Can you work these out from the model? Positions are in its coordinate system, mm. Coordinates: 2 decimals unless noted, no trailing zeros. Loops run counter-clockwise (first coordinate to the right, second up) from the corner with the lowest first, then second, coordinate; pieces in that order, holes last. Notation, with made-up numbers: M 33.5,-22 L 81.5,-22 A25 ccw 81.5,17 Z; hole C -2.75,35 d9. An arc over 180 degrees is marked long. Answer as a JSON object with one key per item and string values. Group by question number.
Item 1: I'm going to push flat-ended pins straight in: pin 1 Ø6 at (x, y) = (-4.5, -21) entering from +Z; pin 2 Ø1.6 at (x, z) = (-6.5, 9.5) entering from +Y; pin 3 Ø3 at (y, z) = (-22.5, 3) entering from +X; pin 4 Ø3 at (y, z) = (10, 6) entering from +X. Where does each tip first touch, or does it pass through?
Item 2: If I drill on line 1 (Z direction, x = -7.5, y = -8); line 2 (Y direction, x = 6, z = 7); line 3 (Y direction, x = 13.25, z = -38.5), over which ranges is the centre line in solid material (lowest first)?
Item 3: Suppose I cut it at C-C (y = 14). Write out the boundary of the cut face in (x, z).
Item 4: Suppose I cut it at B-B (x = -10.5). Write out the boundary of the cut face in (y, z), then the cut area to 3 significant figures.
Item 5: Suppose I cut it at A-A (z = 2). Write out the boundary of the cut face in (x, y), then the cut area to 3 significant figures.
```python
from build123d import *

# Parameters (mm, degrees)
SKETCH1_W           = 29
SKETCH1_H           = 58
BOSS_EXTRUDE1_DEPTH = 57
SKETCH1_3_W         = 1.45
SKETCH1_3_H         = 6.26
BOSS_EXTRUDE2_DEPTH = 16.51
FILLET1_R           = 2
SKETCH2_R           = 0.882124602
BOSS_EXTRUDE3_DEPTH = 16.51
SKETCH2_3_R         = 1.888458119
SKETCH2_3_R_2       = 0.882124602
BOSS_EXTRUDE4_DEPTH = 8
FILLET2_R           = 1


with BuildPart() as part:
    # Sketch1 → Boss-Extrude1 (new body)
    with BuildSketch(Plane.XY):
        Rectangle(SKETCH1_W, SKETCH1_H)
    extrude(amount=-BOSS_EXTRUDE1_DEPTH)

    # Sketch1_3 → Boss-Extrude2 (add)
    with BuildSketch(Plane.XY):
        with Locations((-6.375, 9.13)):
            Rectangle(SKETCH1_3_W, SKETCH1_3_H)
        with Locations((6.375, 9.13)):
            Rectangle(SKETCH1_3_W, SKETCH1_3_H)
    extrude(amount=BOSS_EXTRUDE2_DEPTH)

    # Fillet1
    fillet1_edges = [part.edges().sort_by_distance(p)[0] for p in [
        (0, 29, -57),
        (-14.5, 0, -57),
        (-6.375, 12.26, 16.51),
        (-6.375, 6, 16.51),
        (0, -29, -57),
        (6.375, 6, 16.51),
        (6.375, 12.26, 16.51),
        (14.5, 0, -57),
        (0, -29, 0),
        (-14.5, 0, 0),
        (0, 29, 0),
        (14.5, 0, 0),
        (14.5, -29, -28.5),
        (-14.5, -29, -28.5),
        (-14.5, 29, -28.5),
        (14.5, 29, -28.5),
    ]]
    fillet(fillet1_edges, radius=FILLET1_R)

    # Sketch2 → Boss-Extrude3 (add)
    with BuildSketch(Plane(origin=(0, 0, -57), x_dir=(-1, 0, 0), z_dir=(0, 0, -1))):
        with Locations(Location((0, 0, 0), (0, 0, 180))):
            Circle(SKETCH2_R)
    extrude(amount=BOSS_EXTRUDE3_DEPTH)

    # Sketch2_3 → Boss-Extrude4 (add)
    with BuildSketch(Plane(origin=(0, 0, -57), x_dir=(-1, 0, 0), z_dir=(0, 0, -1))):
        with Locations(Location((0, 0, 0), (0, 0, 180))):
            Circle(SKETCH2_3_R)
        Circle(SKETCH2_3_R_2, mode=Mode.SUBTRACT)
    extrude(amount=BOSS_EXTRUDE4_DEPTH)

    # Fillet2
    fillet2_edges = [part.edges().sort_by_distance(p)[0] for p in [
        (-1.888458119, 0, -65),
    ]]
    fillet(fillet2_edges, radius=FILLET2_R)


solid = part.part
```
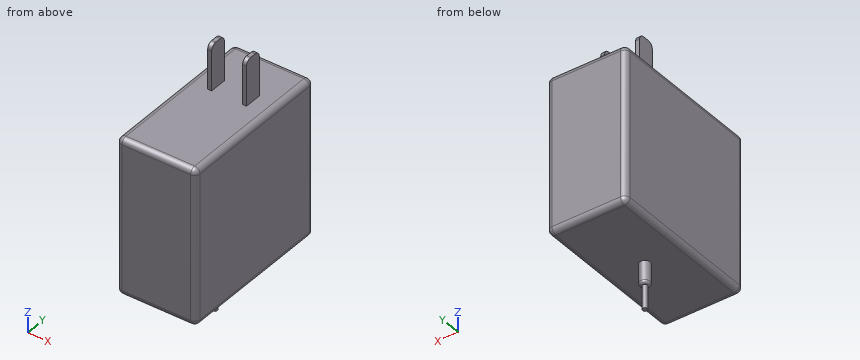
From the geometry:
{
 "1": {"pin 1": "z = 0", "pin 2": "y = 12.26", "pin 3": "through", "pin 4": "x = 7.1"},
 "2": {"line 1": "-57 to 0", "line 2": "6 to 12.26", "line 3": "-28.85 to 28.85"},
 "3": {"outline": "M -14.5,-55 A2 ccw -12.5,-57 L 12.5,-57 A2 ccw 14.5,-55 L 14.5,-2 A2 ccw 12.5,0 L -12.5,0 A2 ccw -14.5,-2 Z"},
 "4": {"outline": "M -29,-55 A2 ccw -27,-57 L 27,-57 A2 ccw 29,-55 L 29,-2 A2 ccw 27,0 L -27,0 A2 ccw -29,-2 Z", "area": "3,300 mm2"},
 "5": {"outline": "M -7.1,6 L -5.65,6 L -5.65,12.26 L -7.1,12.26 Z; M 5.65,6 L 7.1,6 L 7.1,12.26 L 5.65,12.26 Z", "area": "18.2 mm2"}
}
